The model under review builds one solid part; all positions refer to its coordinate system, in mm. A direction names the side the tool comes from. Coordinates: 2 decimals unless noted, no trailing zeros. Order: outer loops, then holes, each group sorted by start corner. A loop starts at its lowest first (then second) coordinate and runs counter-clockwise, first axis right, second up.
from build123d import *

# Parameters (mm, degrees)
F1_DEPTH       = 40
F2_W           = 100
F2_H           = 200
F3_DEPTH       = 100
F4_R           = 5
F5_T           = -2.5
F6_R           = 3
F7_DEPTH       = 25
F8_R           = 8
F9_DEPTH       = 25
F10_R          = 5.5
F11_DEPTH      = 25
F12_R          = 3
F12_R_2        = 1.25
F13_DEPTH      = 10
F14_R          = 3
F15_DEPTH      = 150
F17_START      = -41.94633
F16_W          = 15
F16_H          = 6
F17_DEPTH      = 208.05367
F18_R          = 1.5
F19_DEPTH      = 12.5
F20_R          = 6
F21_DEPTH      = 0.01
F21_DEPTH_BACK = 10
F22_R          = 3
F23_DEPTH      = 12.5
F24_R          = 2
F26_DEPTH      = 150


with BuildPart() as f1:
    # F0 (on Top) → F1 (new body)
    with BuildSketch(Plane.XY):
        with BuildLine():
            Line((-125, 66.5063509461), (-125, -50))
            Line((-125, -50), (125, -50))
            Line((125, -50), (125, 66.5063509461))
            ThreePointArc((125, 66.5063509461), (64.7047614336, 91.4814565299), (3.27e-07, 100))
            ThreePointArc((3.27e-07, 100), (-64.7047611177, 91.4814566146), (-125, 66.5063509461))
        make_face()
    extrude(amount=F1_DEPTH)

    # F2 (on Top) → F3 (cut)
    with BuildSketch(Plane.XY):
        with Locations((-150, -100)):
            Rectangle(F2_W, F2_H)
        with Locations((150, -100)):
            Rectangle(F2_W, F2_H)
    extrude(amount=F3_DEPTH, mode=Mode.SUBTRACT)

    # F4
    f4_edges = [f1.edges().sort_by_distance(p)[0] for p in [
        (-125, 66.506351, 20),
        (125, 66.506351, 20),
        (125, 0, 20),
        (100, 0, 20),
        (-125, 0, 20),
        (-100, 0, 20),
    ]]
    fillet(f4_edges, radius=F4_R)

    # F5
    f5_openings = [f1.faces().sort_by_distance(p)[0] for p in [
        (0, 23.401227, 40),
        (0, -50, 20),
    ]]
    offset(amount=F5_T, openings=f5_openings)

    # F6 (on Top) → F7 (cut)
    with BuildSketch(Plane.XY):
        with Locations((-55.8614357137, -24.1385642863)):
            Circle(F6_R)
        with Locations((55.8614357137, -24.1385642863)):
            Circle(F6_R)
    extrude(amount=F7_DEPTH, mode=Mode.SUBTRACT)

    # F8 (on Top) → F9 (join)
    with BuildSketch(Plane.XY):
        with Locations((-110, 50)):
            Circle(F8_R)
        with Locations((110, 50)):
            Circle(F8_R)
    extrude(amount=F9_DEPTH)

    # F10 (on Top) → F11 (cut)
    with BuildSketch(Plane.XY):
        with Locations((-110, 50)):
            Circle(F10_R)
        with Locations((110, 50)):
            Circle(F10_R)
    extrude(amount=F11_DEPTH, mode=Mode.SUBTRACT)

    # F12 (on Top) → F13 (join)
    with BuildSketch(Plane.XY):
        with Locations((-55, 15)):
            Circle(F12_R)
        with Locations((-55, 15)):
            Circle(F12_R_2, mode=Mode.SUBTRACT)
        with Locations((-39.8, 65.8)):
            Circle(F12_R)
        with Locations((-39.8, 65.8)):
            Circle(F12_R_2, mode=Mode.SUBTRACT)
        with Locations((-11.9, 65.8)):
            Circle(F12_R)
        with Locations((-11.9, 65.8)):
            Circle(F12_R_2, mode=Mode.SUBTRACT)
        with Locations((-6.8, 13.7)):
            Circle(F12_R)
        with Locations((-6.8, 13.7)):
            Circle(F12_R_2, mode=Mode.SUBTRACT)
    extrude(amount=F13_DEPTH)

    # F14 (on Front) → F15 (cut, symmetric)
    with BuildSketch(Plane.XZ):
        with Locations((47, 14)):
            Circle(F14_R)
        with Locations((-47, 14)):
            Circle(F14_R)
    extrude(amount=F15_DEPTH, both=True, mode=Mode.SUBTRACT)

    # F16 (on Front) → F17 (cut)
    with BuildSketch(Plane.XZ.offset(F17_START)):
        with Locations((0, 5.5)):
            Rectangle(F16_W, F16_H)
    extrude(amount=-F17_DEPTH, mode=Mode.SUBTRACT)

    # F18 (on Top) → F19 (cut, symmetric)
    with BuildSketch(Plane.XY):
        with Locations((-3, 95)):
            Circle(F18_R)
        with Locations((3, 95)):
            Circle(F18_R)
    extrude(amount=F19_DEPTH, both=True, mode=Mode.SUBTRACT)

    # F20 (on Top) → F21 (join, two sides)
    with BuildSketch(Plane.XY) as f21_sk:
        with Locations((-35, 90)):
            Circle(F20_R)
        with Locations((35, 90)):
            Circle(F20_R)
    extrude(amount=-F21_DEPTH)
    extrude(f21_sk.sketch, amount=F21_DEPTH_BACK)

    # F22 (on face) → F23 (cut, symmetric)
    with BuildSketch(Plane(origin=(0, 0, 0), x_dir=(1, 0, 0), z_dir=(0, 0, -1))):
        with Locations((-35, -90)):
            Circle(F22_R)
        with Locations((35, -90)):
            Circle(F22_R)
    extrude(amount=F23_DEPTH, both=True, mode=Mode.SUBTRACT)

    # F24
    f24_edges = [f1.edges().sort_by_distance(p)[0] for p in [
        (-32.339812, 95.378048, 6.25),
        (-39.085326, 94.394328, 6.25),
        (39.085326, 94.394328, 6.25),
        (32.339812, 95.378048, 6.25),
        (-118, 50, 2.5),
        (102, 50, 2.5),
    ]]
    fillet(f24_edges, radius=F24_R)

    # F25 (on Right) → F26 (cut, symmetric)
    with BuildSketch(Plane.YZ):
        with BuildLine():
            Line((40, 20), (40, 30))
            ThreePointArc((40, 30), (35, 25), (40, 20))
        make_face()
        with BuildLine():
            ThreePointArc((65, 25), (63.5355339059, 28.5355339059), (60, 30))
            Line((60, 30), (60, 20))
            ThreePointArc((60, 20), (63.5355339059, 21.4644660941), (65, 25))
        make_face()
        with BuildLine():
            Line((60, 30), (40, 30))
            ThreePointArc((40, 30), (43.5355339059, 28.5355339059), (45, 25))
            ThreePointArc((45, 25), (43.5355339059, 21.4644660941), (40, 20))
            Line((40, 20), (60, 20))
            ThreePointArc((60, 20), (55, 25), (60, 30))
        make_face()
        with BuildLine():
            ThreePointArc((45, 25), (43.5355339059, 28.5355339059), (40, 30))
            Line((40, 30), (40, 20))
            ThreePointArc((40, 20), (43.5355339059, 21.4644660941), (45, 25))
        make_face()
        with BuildLine():
            Line((60, 20), (60, 30))
            ThreePointArc((60, 30), (55, 25), (60, 20))
        make_face()
    extrude(amount=F26_DEPTH, both=True, mode=Mode.SUBTRACT)


solid = f1.part
(1) Consider section B-B (x = 47). Give the boundary of the cut face in (y, z).
(2) Wall thickness on line 1 (X direction, y = 50, z = 8.5); line 2 (X direction, y = 18.5, z = 3); line 3 (Y direction, x = -35, z = 4.25): over which ranges is each line inside the solid? List them lowest first.
(3) Consider section C-C (x = -83). Give the boundary of the cut face in (y, z), then the cut area to 3 significant figures.
(4) The part is to be moulded in two halves that separate along X. For faces 4 (the face through (124, 2, 20)), 5 (the face through (-124, 2, 20)), 6 (the face through (-122.5, 35, 21)), say which applies: +X half, -X half, draft (parallel to the pull), parting line (faces both ways), or undercut.
(5) Consider section A-A (y = -12.5). Give the boundary of the cut face in (x, z), then the cut area to 4 significant figures.
(6) Consider section D-D (x = -18.5). Give the boundary of the cut face in (y, z), then the cut area to 3 significant figures.
(7) Insertion check: pin 1 Ø3.5 at (x, y) = (-33.5, 91.5) entering from +Z; pin 2 Ø6 at (x, z) = (-47.5, 6.5) entering from +Y; pin 3 Ø2 at (x, y) = (-55, 15) entering from +Z; pin 4 Ø2.5 at (x, y) = (-3, 95) entering from +Z. Each pin has a flat end and moves straight along its axis. Give the tip position at first contact, or say it passes through.
(8) Tool access review of faces 1 (the face through (-115.495, 50.242, 9.86)), 2 (the face through (-97.5, -28, 21)), 3 (the face through (-5.19, 16.23, 6.2)): name each direction out of +Z, -Z, +X, -X, +Y, -Y from which nothing blocks a thin tool from reaching the whole face with its end or side.
Findings:
1. outline: (-50, 0) - (95.54, 0) - (95.54, 11) - (93, 11) - (93, 2.5) - (-50, 2.5) - close; (93, 17) - (95.54, 17) - (95.54, 40) - (93, 40) - close
2. line 1: x = -125 to -122.5, -118 to -115.5, -104.5 to -102, 102 to 104.5, 115.5 to 118, 122.5 to 125
2. line 2: x = -125 to -122.5, 122.5 to 125
2. line 3: y = 84 to 87, 93 to 97.54
3. outline: (-50, 0) - (85.82, 0) - (85.82, 40) - (83.17, 40) - (83.17, 2.5) - (-50, 2.5) - close
3. area: 439 mm2
4. face 4: +X half
4. face 5: -X half
4. face 6: undercut
5. outline: (-100, 0) - (100, 0) - (100, 40) - (97.5, 40) - (97.5, 2.5) - (-97.5, 2.5) - (-97.5, 40) - (-100, 40) - close
5. area: 687.5 mm2
6. outline: (-50, 0) - (99.31, 0) - (99.31, 40) - (96.81, 40) - (96.81, 2.5) - (-50, 2.5) - close
6. area: 467 mm2
7. pin 1: stops at z = 10
7. pin 2: stops at y = 96.01
7. pin 3: stops at z = 2.5
7. pin 4: passes through
8. face 1: +Z, -Z
8. face 2: +Z, -Y
8. face 3: +Z
